Design review of the part built by this model. Coordinates are the model's own, in mm. Coordinates: 2 decimals unless noted, no trailing zeros. Loops run counter-clockwise (first coordinate to the right, second up) from the corner with the lowest first, then second, coordinate; pieces in that order, holes last. Notation, with made-up numbers: (-9, 26) - (8, 26) arc R16 cw to (8, 41) - close; hole circle Ø2 at (41, 22). An arc over 180 degrees is marked (long way). Return JSON: item names as keys, results as strings. Group by question number.
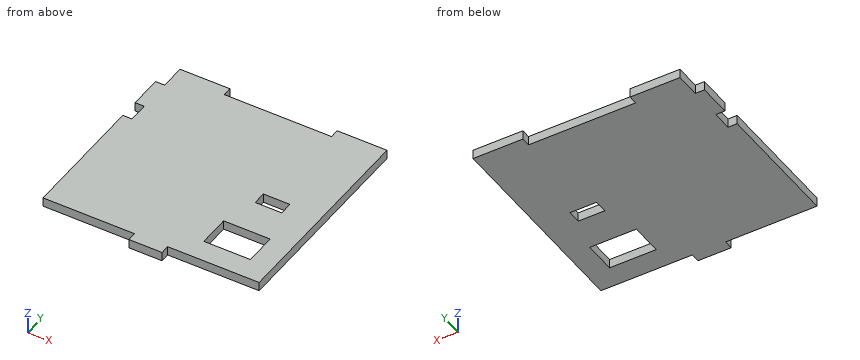
from build123d import *

# Parameters (mm, degrees)
CROQUIS1_W              = 28
CROQUIS1_H              = 19.35
CROQUIS1_W_2            = 16
CROQUIS1_H_2            = 8
SALIENTE_EXTRUIR1_DEPTH = 5.5


with BuildPart() as part:
    # Croquis1 → Saliente-Extruir1 (new body)
    with BuildSketch(Plane.XY):
        Polygon((468.016438709, 88.608229285), (468.016438709, -36.391770715), (413.016438709, -36.391770715), (413.016438709, -41.891770715), (393.016438709, -41.891770715), (393.016438709, -36.391770715), (338.016438709, -36.391770715), (338.016438709, 41.608229285), (343.516438709, 41.608229285), (343.516438709, 53.608229285), (338.016438709, 53.608229285), (338.016438709, 73.608229285), (343.516438709, 73.608229285), (343.516438709, 88.608229285), (373.516438709, 88.608229285), (373.516438709, 83.108229285), (438.016438709, 83.108229285), (438.016438709, 88.608229285), align=None)
        with Locations((440.516438709, -13.325)):
            Rectangle(CROQUIS1_W, CROQUIS1_H, mode=Mode.SUBTRACT)
        with Locations((440.516438709, 21.433223203)):
            Rectangle(CROQUIS1_W_2, CROQUIS1_H_2, mode=Mode.SUBTRACT)
    extrude(amount=SALIENTE_EXTRUIR1_DEPTH)


solid = part.part
Item 1: Add section C-C (z = 2). State the section outline as (x, y) points, then the cut area to 3 significant figures.
Item 2: Add section B-B (y = -7). State the section outline as (x, z) points, then the cut area to 3 significant figures.
Item 3: To check wall thickness, follow line 1 (Y direction, x = 445.5, z = 1.1); line 2 (X direction, y = 20, z = 1.8); line 3 (Y direction, x = 434, z = 3). State the ranges of each line that lie inside material, in increasing order. Write a range as from..to.
Item 4: Add section D-D (x = 428.5). State the section outline as (y, z) points, then the cut area to 3 significant figures.
Item 5: For P1, Ø3, axis at x = 339.5, z = 2.5, coming from the +Y side; P2, Ø1.6, axis at y = 85, z = 3, coming from the -X side; P3, Ø3, axis at x = 358.5, z = 3, coming from the -Y side, all flat-tipped, find the tip position at first contact; note any pin that passes through.
Item 6: Add section A-A (x = 445.5). State the section outline as (y, z) points.
Answers below:
{
 "1": {"outline": "(338.02, -36.39) - (393.02, -36.39) - (393.02, -41.89) - (413.02, -41.89) - (413.02, -36.39) - (468.02, -36.39) - (468.02, 88.61) - (438.02, 88.61) - (438.02, 83.11) - (373.52, 83.11) - (373.52, 88.61) - (343.52, 88.61) - (343.52, 73.61) - (338.02, 73.61) - (338.02, 53.61) - (343.52, 53.61) - (343.52, 41.61) - (338.02, 41.61) - close; hole (426.52, -23) - (454.52, -23) - (454.52, -3.65) - (426.52, -3.65) - close; hole (432.52, 17.43) - (448.52, 17.43) - (448.52, 25.43) - (432.52, 25.43) - close", "area": "15,200 mm^2"},
 "2": {"outline": "(338.02, 0) - (426.52, 0) - (426.52, 5.5) - (338.02, 5.5) - close; (454.52, 0) - (468.02, 0) - (468.02, 5.5) - (454.52, 5.5) - close", "area": "561 mm^2"},
 "3": {"line 1": "y = -36.39..-23, -3.65..17.43, 25.43..88.61", "line 2": "x = 338.02..432.52, 448.52..468.02", "line 3": "y = -36.39..-23, -3.65..17.43, 25.43..83.11"},
 "4": {"outline": "(-36.39, 0) - (-23, 0) - (-23, 5.5) - (-36.39, 5.5) - close; (-3.65, 0) - (83.11, 0) - (83.11, 5.5) - (-3.65, 5.5) - close", "area": "551 mm^2"},
 "5": {"P1": "stops at y = 73.61", "P2": "stops at x = 343.52", "P3": "stops at y = -36.39"},
 "6": {"outline": "(-36.39, 0) - (-23, 0) - (-23, 5.5) - (-36.39, 5.5) - close; (-3.65, 0) - (17.43, 0) - (17.43, 5.5) - (-3.65, 5.5) - close; (25.43, 0) - (88.61, 0) - (88.61, 5.5) - (25.43, 5.5) - close"}
}
